from build123d import *

# Parameters (mm, degrees)
CROQUIS1_W              = 50.8
CROQUIS1_H              = 6.31
SALIENTE_EXTRUIR1_DEPTH = 285.44
CROQUIS3_W              = 50.8
CROQUIS3_H              = 6.31
SALIENTE_EXTRUIR2_DEPTH = 544.51
CROQUIS4_W              = 50.8
CROQUIS4_H              = 6.31
CROQUIS5_W              = 50.8
CROQUIS5_H              = 68
CORTAR_EXTRUIR1_DEPTH   = 10
CROQUIS11_W             = 48.12
CROQUIS11_H             = 211.5
CORTAR_EXTRUIR2_DEPTH   = 50.8


with BuildPart() as part:
    # Croquis1 → Saliente-Extruir1 (new body)
    with BuildSketch(Plane.XY):
        Rectangle(CROQUIS1_W, CROQUIS1_H)
    extrude(amount=SALIENTE_EXTRUIR1_DEPTH)

    # Croquis3 → Saliente-Extruir2 (add)
    with BuildSketch(Plane.XZ.offset(3.155)):
        with Locations((0, 3.155)):
            Rectangle(CROQUIS3_W, CROQUIS3_H)
    extrude(amount=-SALIENTE_EXTRUIR2_DEPTH)

    # Barrer1: sweep along a curve in space
    with BuildLine() as barrer1_path:
        Line((0, 541.355, 3.155), (0, 551.355, 3.155))
        Line((0, 551.355, 3.155), (0, 551.355, 44.965))
        Line((0, 551.355, 44.965), (0, 634.515, 44.965))
    # Croquis4 → Barrer1 (sweep)
    with BuildSketch(Plane(origin=(0, 541.355, 0), x_dir=(1, 0, 0), z_dir=(0, 1, 0))):
        with Locations((0, -3.155)):
            Rectangle(CROQUIS4_W, CROQUIS4_H)
    sweep(path=barrer1_path.line, transition=Transition.RIGHT)

    # Croquis5 → Cortar-Extruir1 (cut)
    with BuildSketch(Plane.XZ.offset(3.155)):
        with Locations((0, 251.44)):
            Rectangle(CROQUIS5_W, CROQUIS5_H)
    extrude(amount=-CORTAR_EXTRUIR1_DEPTH, mode=Mode.SUBTRACT)

    # Croquis11 → Cortar-Extruir2 (cut)
    with BuildSketch(Plane(origin=(25.4, 0, 0), x_dir=(0, 0, -1), z_dir=(1, 0, 0))):
        with Locations((-24.06, 528.765)):
            Rectangle(CROQUIS11_W, CROQUIS11_H)
    extrude(amount=-CORTAR_EXTRUIR2_DEPTH, mode=Mode.SUBTRACT)


solid = part.part
The listing builds one solid part. Answer for the finished solid, in the listing's coordinates (mm). A direction names the side the tool comes from. Give positions to 0.01 mm unless a question says otherwise; leave off trailing zeros. Write each loop counter-clockwise with the first axis right and the second up, starting at its lowest first coordinate (ties: lowest second). Pieces come first, ordered by that corner, then holes.
Item 1: Find the intervals of material crossed by line 1 along Y through (x, z) = (19, 49.5) (3 decimals); line 2 along Z through (x, y) = (-17, 66), in increasing order.
Item 2: A flat-ended cylindrical pin translates along its axis: P1, Ø10, axis at x = 18.5, y = 238.5, coming from the +Z side. Find the tip coordinate at first contact, or state that the pin passes through.
Item 3: Section C-C, the plane y = 143.5 is taken. Write down the section's boundary in (x, z).
Item 4: Section A-A, the plane x = 12.5 is taken. Write down the section's boundary in (y, z) (3 decimals).
Item 5: Section B-B, the plane z = 90 is taken. Write down the section's boundary in (x, y) (3 decimals), plus the area to 3 significant figures.
Item 6: Which of the six approach directions +Z, -Z, +X, -X, +Y, -Y give full straight-line access (tool end or side, diameter ignored) to faces 1 (the flat face through (0, -3.155, 107)), 2 (the flat face through (0, 3.155, 110))?
Completed:
1. line 1: y = -3.155 to 3.155
1. line 2: z = 0 to 6.31
2. P1: stops at z = 6.31
3. outline: (-25.4, 0) - (25.4, 0) - (25.4, 6.31) - (-25.4, 6.31) - close
4. outline: (-3.155, 0) - (423.015, 0) - (423.015, 6.31) - (3.155, 6.31) - (3.155, 217.44) - (-3.155, 217.44) - close
5. outline: (-25.4, -3.155) - (25.4, -3.155) - (25.4, 3.155) - (-25.4, 3.155) - close
5. area: 321 mm2
6. face 1: +Z, -Z, +X, -X, -Y
6. face 2: +Z, +X, -X, +Y
